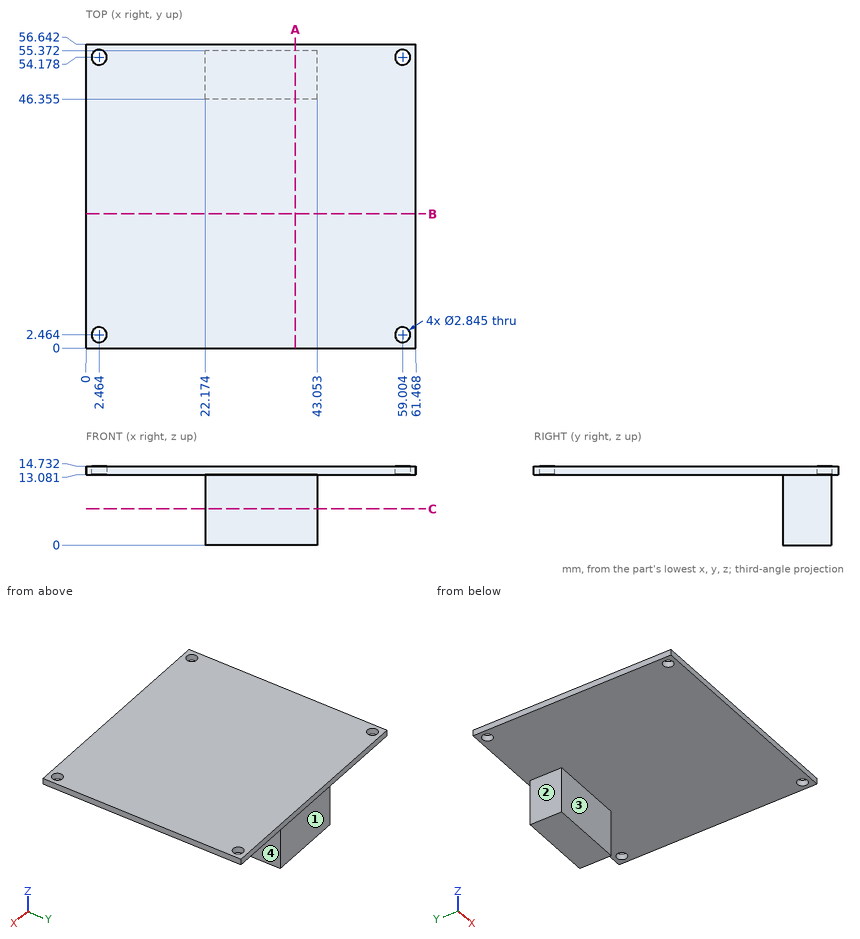
Check sheet for the drawn part. Datum: minimum x, y, z corner. Units: mm. A direction names the side the tool comes from. Round coordinates to 2 decimals unless told otherwise and drop trailing zeros. Order: outer loops, then holes, each group sorted by start corner. A loop starts at its lowest first (then second) coordinate and runs counter-clockwise, first axis right, second up. Notation, with made-up numbers: M 9,-38 L 58,-38 A13 cw 58,-20 Z; hole C 53.25,23.25 d10. An arc over 180 degrees is marked long. Write each question's results on one line, items separated by ' | '. Start each with the question number.
1. Cross-section at A-A on x = 39. Record the boundary of the cut face in (y, z) (3 decimals).
2. Material ranges on L1, parallel to Y at x = 32, z = 11.25 (3 decimals); L2, parallel to Z at x = 3, y = 12, recorded low to high. Write a range as from..to.
3. Go/stop test with flat-tipped pins: P1, Ø3, axis at y = 47.5, z = 11.5, coming from the -X side; P2, Ø8, axis at y = 46, z = 4, coming from the +X side; P3, Ø17, axis at x = 24, y = 31, coming from the -Z side. Record where each tip stops, or that it passes through.
4. Set-up check for the marked faces 1, 2, 3 and 4: record each of +Z, -Z, +X, -X, +Y, -Y from which the full face is reachable in a straight line by a thin tool's end or side.
5. Cross-section at C-C on z = 6.75. Record the boundary of the cut face in (x, y) (1 decimal).
6. Cross-section at B-B on y = 25. Record the boundary of the cut face in (x, z).
Resolved:
1) outline: M 0,13.081 L 46.355,13.081 L 46.355,0 L 55.372,0 L 55.372,13.081 L 56.642,13.081 L 56.642,14.732 L 0,14.732 Z
2) L1: 46.355..55.372 | L2: 13.08..14.73
3) P1: x = 22.17 | P2: x = 43.05 | P3: z = 13.08
4) face 1: -Z, +X, -X, +Y | face 2: -Z, -X, +Y, -Y | face 3: -Z, +X, -X, -Y | face 4: -Z, +X, +Y, -Y
5) outline: M 22.2,46.4 L 43.1,46.4 L 43.1,55.4 L 22.2,55.4 Z
6) outline: M 0,13.08 L 61.47,13.08 L 61.47,14.73 L 0,14.73 Z
